Design review of the part built by this model. Coordinates are the model's own, in mm. Face numbers are marked on the shaded views. A direction names the side the tool comes from. Give positions to 0.01 mm unless a question says otherwise; leave off trailing zeros. Loops run counter-clockwise (first coordinate to the right, second up) from the corner with the lowest first, then second, coordinate; pieces in that order, holes last. Notation, with made-up numbers: M -17.75,72.5 L 18.25,72.5 A9 cw 18.25,87.5 Z; hole C -28,27.5 d4. An arc over 180 degrees is marked long. Use a Markdown table: item, result. Add a question column.
(1) Draft analysis for pull direction Y (two halves, no side actions). For the marked faces 1, 2 and 3, state which applies: pulls with the +Y half, pulls with the -Y half, needs draft (parallel to the pull), parting line crosses it, or undercut.
(2) For probe 1 along X at (y, z) = (37, 82); probe 2 along Y at (x, z) = (102.5, 68); probe 3 along Z at (x, y) = (332.5, 45), list the stretches that pass through material, from the lowest coordinate up.
(3) Add section D-D, the plane z = 126.5. Give the boundary of the cut face in (x, y).
(4) Add section B-B, the plane x = 326. Give the boundary of the cut face in (y, z).
(5) For the marked faces 4 and 5, list the 3-axis set-ups (+Z, -Z, +X, -X, +Y, -Y) from which the entire face can be reached by the end or side of a thin tool; tool diameter is ignored.
(6) Insertion check: pin 1 Ø1 at (y, z) = (9.5, 109.5) entering from -X; pin 2 Ø3 at (x, y) = (118.5, 34) entering from +Z; pin 3 Ø2 at (y, z) = (12, 44) entering from +X. Each pin has a flat end and moves straight along its axis. Give the tip position at first contact, or say it passes through.
(7) Add section C-C, the plane z = 323. Give the boundary of the cut face in (x, y).
(8) Add section A-A, the plane y = 5. Give the boundary of the cut face in (x, z).
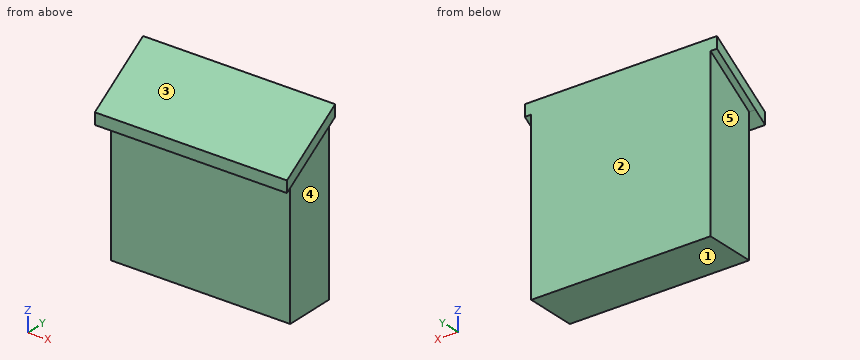
```python
from build123d import *

# Parameters (mm, degrees)
F1_DEPTH = 355.6
F3_DEPTH = 12.7
F5_DEPTH = 12.7


with BuildPart() as f1:
    # F0 (on Right) → F1 (new body)
    with BuildSketch(Plane.YZ):
        Polygon((0, 266.650707), (0, 0), (101.6, 0), (101.6, 355.6), (-25.4, 272.836097), (-25.4, 250.097926), align=None)
    extrude(amount=F1_DEPTH)

    # F2 (on face) → F3 (join)
    with BuildSketch(Plane.YZ.offset(355.6)):
        Polygon((-25.4, 250.097926), (0, 266.650707), (101.6, 332.861829), (101.6, 355.6), (-25.4, 272.836097), align=None)
    extrude(amount=F3_DEPTH)

    # F4 (on face) → F5 (join)
    with BuildSketch(Plane(origin=(0, 0, 0), x_dir=(0, -1, 0), z_dir=(-1, 0, 0))):
        Polygon((-101.6, 332.861829), (0, 266.650707), (25.4, 250.097926), (25.4, 272.836097), (-101.6, 355.6), align=None)
    extrude(amount=F5_DEPTH)


solid = f1.part
```
Established:
| question | item | result |
|---|---|---|
| 1 | face 1 | needs draft |
| 1 | face 2 | pulls with the +Y half |
| 1 | face 3 | pulls with the -Y half |
| 2 | probe 1 | 0 to 355.6 |
| 2 | probe 2 | 0 to 101.6 |
| 2 | probe 3 | 0 to 318.71 |
| 3 | outline | M 0,0 L 355.6,0 L 355.6,101.6 L 0,101.6 Z |
| 4 | outline | M -25.4,250.1 L 0,266.65 L 0,0 L 101.6,0 L 101.6,355.6 L -25.4,272.84 Z |
| 5 | face 4 | -Z, +X, +Y |
| 5 | face 5 | -Z, -X, +Y |
| 6 | pin 1 | x = 0 |
| 6 | pin 2 | z = 312.52 |
| 6 | pin 3 | x = 355.6 |
| 7 | outline | M -12.7,51.58 L 368.3,51.58 L 368.3,86.47 L 355.6,86.47 L 355.6,101.6 L 0,101.6 L 0,86.47 L -12.7,86.47 Z |
| 8 | outline | M -12.7,269.91 L 0,269.91 L 0,0 L 355.6,0 L 355.6,269.91 L 368.3,269.91 L 368.3,292.65 L -12.7,292.65 Z |
